from build123d import *

# Parameters (mm, degrees)
REVOLVE1_ANGLE            = 180
TAP_DRILL_FOR_4_40_TAP1_D = 2.2606
CIRPATTERN1_COUNT         = 12


with BuildPart() as part:
    # Sketch1 → Revolve1 (revolve)
    with BuildSketch(Plane.XY):
        Polygon((56.388, 0), (56.388, 9.525), (47.625, 9.525), (47.625, 15.875), (88.9, 15.875), (88.9, -15.875), (47.625, -15.875), (47.625, -9.525), (56.388, -9.525), align=None)
    revolve(axis=Axis((0, 22.539286723, 0), (0, -1, 0)), revolution_arc=REVOLVE1_ANGLE)

    # Tap Drill for #4-40 Tap1 (through all)
    with Locations(Plane(origin=(49.878671003, 15.875, 13.364949615), x_dir=(0, 0, 1), z_dir=(0, 1, 0))):
        with Locations((0, 0)):
            tap_drill_for_4_40_tap1 = Hole(TAP_DRILL_FOR_4_40_TAP1_D / 2)

    # CirPattern1: Tap Drill for #4-40 Tap1 ×12 about axis, 6 skipped
    cirpattern1_axis = Axis((0, 15.875, 0), (0, 1, 0))
    add([tap_drill_for_4_40_tap1.rotate(cirpattern1_axis, i * 360 / CIRPATTERN1_COUNT) for i in range(1, CIRPATTERN1_COUNT) if i not in (1, 2, 3, 4, 5, 6)], mode=Mode.SUBTRACT)


solid = part.part
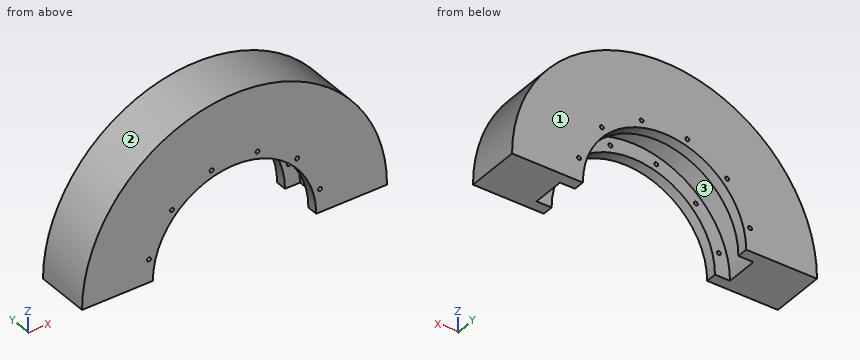
Can you work these out from the model? Positions are in its coordinate system, mm. Face numbers are marked on the shaded views. Give positions to 0.01 mm unless a question says otherwise; leave off trailing zeros. Loops run counter-clockwise (first coordinate to the right, second up) from the corner with the lowest first, then second, coordinate; pieces in that order, holes last. Notation, with made-up numbers: (10, 3) -> (56, 3) arc R14 cw to (56, 26) -> close; hole circle Ø4 at (-38, 76). An arc over 180 degrees is marked (long way). Return JSON: item names as keys, results as strings.
Q1. I want a section at C-C, the plane z = 27. List the corners of the cut face in (x, y) for me (3 decimals), then the cut area to 3 significant figures.
Checks:
{"outline": "(-84.701, -15.875) -> (-39.232, -15.875) -> (-39.232, -9.525) -> (-49.504, -9.525) -> (-49.504, 9.525) -> (-39.232, 9.525) -> (-39.232, 15.875) -> (-84.701, 15.875) -> close; (39.232, -15.875) -> (84.701, -15.875) -> (84.701, 15.875) -> (39.232, 15.875) -> (39.232, 9.525) -> (49.504, 9.525) -> (49.504, -9.525) -> (39.232, -9.525) -> close", "area": "2,500 mm2"}
Q2. I want a section at A-A, the plane y = 12. List the corners of the cut face in (x, z) for me (3 decimals), then the cut area to 3 significant figures.
Checks:
{"outline": "(-88.9, 0) -> (-47.625, 0) arc R47.625 cw to (47.625, 0) -> (88.9, 0) arc R88.9 ccw to start; hole circle Ø2.261 at (-49.879, 13.365); hole circle Ø2.261 at (-36.514, 36.514); hole circle Ø2.261 at (-13.365, 49.879); hole circle Ø2.261 at (13.365, 49.879); hole circle Ø2.261 at (36.514, 36.514); hole circle Ø2.261 at (49.879, 13.365)", "area": "8,830 mm2"}
Q3. For pin 1 Ø1.8 at (x, z) = (-13.36, 49.88) entering from +Y; pin 2 Ø2.5 at (x, z) = (-36.51, 36.51) entering from -Y (3 decimals); pin 3 Ø8 at (y, z) = (-3, 11.5) entering from -X; pin 4 Ø5 at (x, y) = (57, -3) entering from +Z, each with a flat end and sliding along its axis, tell me the tip position at first contact or that it passes through.
Checks:
{"pin 1": "passes through", "pin 2": "stops at y = -15.875", "pin 3": "stops at x = -88.58", "pin 4": "stops at z = 70.24"}
Q4. I want a section at B-B, the plane x = 0. List the corners of the cut face in (y, z) for me (3 decimals), then the cut area to 3 significant figures.
Checks:
{"outline": "(-15.875, 47.625) -> (-9.525, 47.625) -> (-9.525, 56.388) -> (9.525, 56.388) -> (9.525, 47.625) -> (15.875, 47.625) -> (15.875, 88.9) -> (-15.875, 88.9) -> close", "area": "1,140 mm2"}
Q5. We'd pull the mould along X, two halves only. Please class the marked faces 1, 2 and 3: released by +X, released by -X, zero draft, split by the parting line, or undercut.
Checks:
{"face 1": "zero draft", "face 2": "split by the parting line", "face 3": "undercut"}
Q6. I need wall thicknesses on probe 1 along X at (y, z) = (12.5, 49); probe 2 along Z at (x, y) = (-1.5, 5.5); probe 3 along Y at (x, z) = (-38.5, 31) (3 decimals). Which ranges of each line are inside material? Lowest first, please.
Checks:
{"probe 1": "x = -74.18 to -14.08, -12.65 to 12.65, 14.08 to 74.18", "probe 2": "z = 56.37 to 88.89", "probe 3": "y = -15.875 to -9.525, 9.525 to 15.875"}
Q7. I want a section at D-D, the plane y = -6. List the corners of the cut face in (x, z) for me, then the cut area to 3 significant figures.
Checks:
{"outline": "(-88.9, 0) -> (-56.39, 0) arc R56.39 cw to (56.39, 0) -> (88.9, 0) arc R88.9 ccw to start", "area": "7,420 mm2"}
